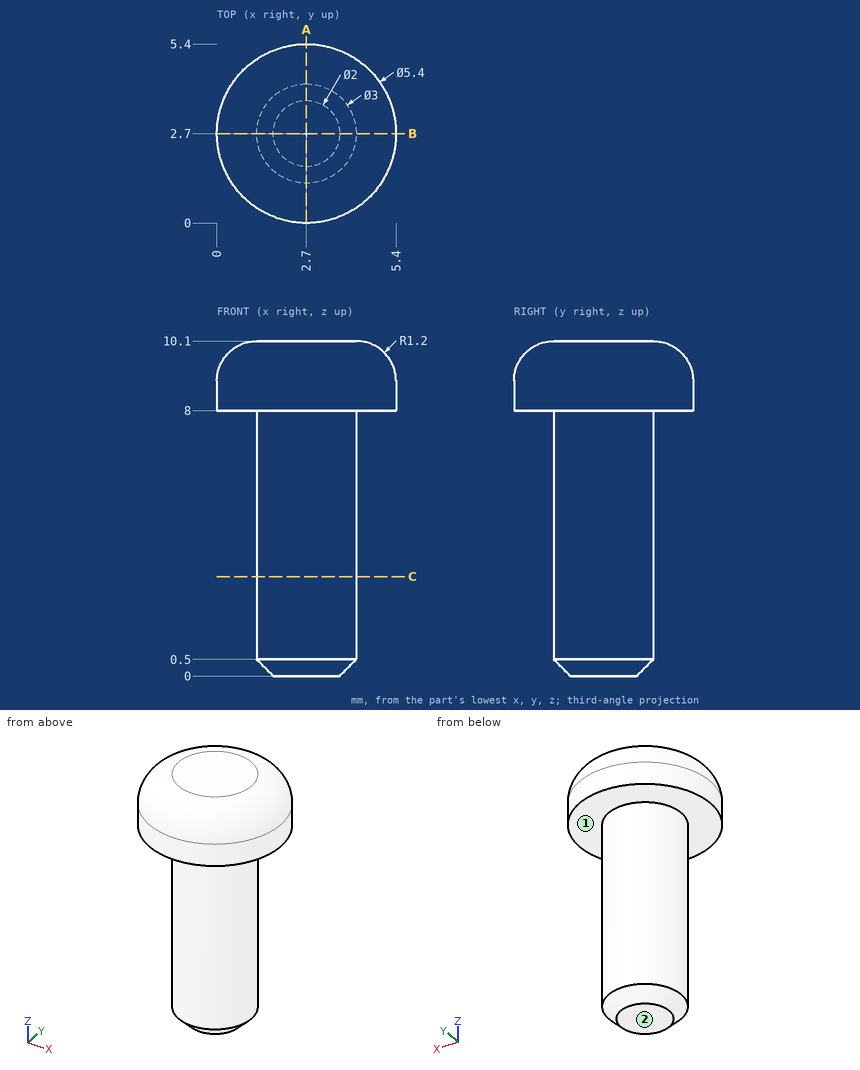
Job drawing, mm, ordinate dimensions from the low corner. One solid piece. A direction names the side the tool comes from. Coordinates: 2 decimals unless noted, no trailing zeros. Write each loop counter-clockwise with the first axis right and the second up, starting at its lowest first coordinate (ties: lowest second). Pieces come first, ordered by that corner, then holes.
Item 1: Slice it at C-C (z = 3). Write the cut outline in (x, y), and give its area (3 significant figures).
Item 2: Pin check, flat tips, straight feed: pin 1 (3 mm diameter, centred on x = 1.5, z = 5.5, fed in from -Y); pin 2 (2 mm diameter, centred on x = 1, y = 2.5, fed in from +Z); pin 3 (1.5 mm diameter, centred on y = 2.5, z = 4, fed in from -X); pin 4 (1 mm diameter, centred on y = 4, z = 6, fed in from +X). Stop position of each tip, or through.
Item 3: Probe line 1 (Z direction, x = 2.5, y = 4.25); line 2 (X direction, y = 4.5, z = 9.5); line 3 (Z direction, x = 4.85, y = 1.35). List the from-to ranges inside material, lowest first.
Item 4: Which spindle directions (+Z, -Z, +X, -X, +Y, -Y) get a long thin tool onto all of the face, cutting with end or side? Do the marked faces 1 and 2. Say none if no direction does.
Item 5: Slice it at A-A (x = 2.7). Write the cut outline in (y, z), and give its area (3 significant figures).
Results found:
1. outline: circle Ø3 at (2.7, 2.7)
1. area: 7.07 mm2
2. pin 1: stops at y = 1.2
2. pin 2: stops at z = 10.1
2. pin 3: stops at x = 1.2
2. pin 4: stops at x = 3.97
3. line 1: z = 8 to 10.1
3. line 2: x = 0.91 to 4.49
3. line 3: z = 8 to 9.5
4. face 1: -Z
4. face 2: -Z, +X, -X, +Y, -Y
5. outline: (0, 8) - (1.2, 8) - (1.2, 0.5) - (1.7, 0) - (3.7, 0) - (4.2, 0.5) - (4.2, 8) - (5.4, 8) - (5.4, 8.9) arc R1.2 ccw to (4.2, 10.1) - (1.2, 10.1) arc R1.2 ccw to (0, 8.9) - close
5. area: 34.5 mm2
